Here's how the part is built. I have some questions about the finished solid (model axes, mm). Face numbers are marked on the shaded views. A direction names the side the tool comes from. Round coordinates to 2 decimals unless told otherwise and drop trailing zeros. Loops run counter-clockwise (first coordinate to the right, second up) from the corner with the lowest first, then second, coordinate; pieces in that order, holes last. Notation, with made-up numbers: (73, -29) -> (132, -29) arc R5 cw to (132, -20) -> close; hole circle Ø10 at (25.5, -23). An arc over 180 degrees is marked (long way). Use CSV: the item, a comma, the result in double quotes. Start each with the question number.
from build123d import *

# Parameters (mm, degrees)
BASE_FLANGE1_DEPTH      = 4.7752
EDGE_FLANGE1_DEPTH      = 50.8
EDGE_FLANGE1_BEND_DEPTH = 50.8
EDGE_FLANGE2_DEPTH      = 57.15
EDGE_FLANGE2_BEND_DEPTH = 57.15
CUT_EXTRUDE1_DEPTH      = 132.397433882
CUT_EXTRUDE1_DEPTH_BACK = 132.397433882
SKETCH18_R              = 5.159375
CUT_EXTRUDE3_DEPTH      = 122.772271015
CUT_EXTRUDE3_DEPTH_BACK = 122.772271015
SKETCH20_R              = 5.159375


# Sheet-metal steps are written as plain solids
with BuildPart() as part:
    # Sketch1 → Base-Flange1 (new body)
    with BuildSketch(Plane(origin=(0, 0, 0), x_dir=(1, 0, 0), z_dir=(0, 1, 0))):
        Polygon((26.9875, -28.575), (26.9875, 28.575), (28.575, 28.575), (28.575, 79.375), (-28.575, 79.375), (-28.575, -79.375), (28.575, -79.375), (28.575, -28.575), align=None)
    extrude(amount=-BASE_FLANGE1_DEPTH)

    # Edge-Flange1 section (across the edge) → Edge-Flange1 (add)
    with BuildSketch(Plane(origin=(34.5186, 0, -28.575), x_dir=(-1, 0, 0), z_dir=(0, 0, -1))):
        with BuildLine():
            Line((-4.7752, 5.9436), (-4.7752, 69.85))
            Line((-4.7752, 69.85), (0, 69.85))
            Line((0, 69.85), (0, 5.9436))
            ThreePointArc((0, 5.9436), (1.740840135, 1.740840135), (5.9436, 0))
            Line((5.9436, 0), (5.9436, -4.7752))
            ThreePointArc((5.9436, -4.7752), (-1.635736166, -1.635736166), (-4.7752, 5.9436))
        make_face()
    extrude(amount=EDGE_FLANGE1_DEPTH)

    # Edge-Flange1 section 2 (across the edge) → Edge-Flange1 bend (add)
    with BuildSketch(Plane(origin=(34.5186, 0, 79.375), x_dir=(-1, 0, 0), z_dir=(0, 0, -1))):
        with BuildLine():
            Line((-4.7752, 5.9436), (-4.7752, 69.85))
            Line((-4.7752, 69.85), (0, 69.85))
            Line((0, 69.85), (0, 5.9436))
            ThreePointArc((0, 5.9436), (1.740840135, 1.740840135), (5.9436, 0))
            Line((5.9436, 0), (5.9436, -4.7752))
            ThreePointArc((5.9436, -4.7752), (-1.635736166, -1.635736166), (-4.7752, 5.9436))
        make_face()
    extrude(amount=EDGE_FLANGE1_BEND_DEPTH)

    # Edge-Flange2 section (across the edge) → Edge-Flange2 (add)
    with BuildSketch(Plane(origin=(28.575, -4.7752, 86.9061), x_dir=(0, 0, -1), z_dir=(-1, 0, 0))):
        with BuildLine():
            Line((-4.7752, 5.9436), (-4.7752, 17.4498))
            Line((-4.7752, 17.4498), (0, 17.4498))
            Line((0, 17.4498), (0, 5.9436))
            ThreePointArc((0, 5.9436), (1.740840135, 1.740840135), (5.9436, 0))
            Line((5.9436, 0), (7.5311, 0))
            Line((7.5311, 0), (7.5311, -4.7752))
            Line((7.5311, -4.7752), (5.9436, -4.7752))
            ThreePointArc((5.9436, -4.7752), (-1.635736166, -1.635736166), (-4.7752, 5.9436))
        make_face()
    extrude(amount=EDGE_FLANGE2_DEPTH)

    # Edge-Flange2 section 2 (across the edge) → Edge-Flange2 bend (add)
    with BuildSketch(Plane(origin=(-28.575, -4.7752, -86.9061), x_dir=(0, 0, 1), z_dir=(1, 0, 0))):
        with BuildLine():
            Line((-4.7752, 5.9436), (-4.7752, 17.4498))
            Line((-4.7752, 17.4498), (0, 17.4498))
            Line((0, 17.4498), (0, 5.9436))
            ThreePointArc((0, 5.9436), (1.740840135, 1.740840135), (5.9436, 0))
            Line((5.9436, 0), (7.5311, 0))
            Line((7.5311, 0), (7.5311, -4.7752))
            Line((7.5311, -4.7752), (5.9436, -4.7752))
            ThreePointArc((5.9436, -4.7752), (-1.635736166, -1.635736166), (-4.7752, 5.9436))
        make_face()
    extrude(amount=EDGE_FLANGE2_BEND_DEPTH)

    # Sketch18 → Cut-Extrude1 (cut, two sides: drawn at the far end of the back side and taken through both)
    with BuildSketch(Plane.ZY.offset(-34.5186).offset(-CUT_EXTRUDE1_DEPTH_BACK)):
        with Locations(Location((-53.975, 50.8, 0), (0, 0, 270))):
            Circle(SKETCH18_R)
        with Locations(Location((-53.975, 19.05, 0), (0, 0, 270))):
            Circle(SKETCH18_R)
        with Locations(Location((53.975, 50.8, 0), (0, 0, 270))):
            Circle(SKETCH18_R)
        with Locations(Location((53.975, 19.05, 0), (0, 0, 270))):
            Circle(SKETCH18_R)
    extrude(amount=CUT_EXTRUDE1_DEPTH + CUT_EXTRUDE1_DEPTH_BACK, mode=Mode.SUBTRACT)

    # Sketch20 → Cut-Extrude3 (cut, two sides: drawn at the far end of the back side and taken through both)
    with BuildSketch(Plane(origin=(0, 0, 0), x_dir=(1, 0, 0), z_dir=(0, 1, 0)).offset(-CUT_EXTRUDE3_DEPTH_BACK)):
        with Locations((-72.900583951, 79.249926239)):
            Circle(SKETCH20_R)
        with Locations(Location((-3.175, 75.082739816, 0), (0, 0, 270))):
            Circle(SKETCH20_R)
        with Locations(Location((-9.236362071, -26.336291386, 0), (0, 0, 270))):
            Circle(SKETCH20_R)
        with Locations((-78.961946022, -22.169104962)):
            Circle(SKETCH20_R)
    extrude(amount=CUT_EXTRUDE3_DEPTH + CUT_EXTRUDE3_DEPTH_BACK, mode=Mode.SUBTRACT)


solid = part.part
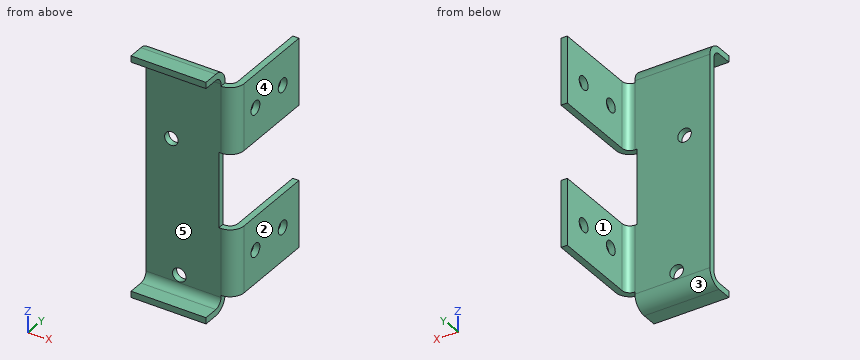
Q1. I want a section at C-C, the plane x = 7.5. List the corners of the cut face in (y, z) for me (1 decimal).
Q2. I want a section at D-D, the plane x = 30.5. List the corners of the cut face in (y, z) for me (3 decimals), then the cut area to 3 significant figures.
Q3. Will these pins go through, and if not, where does the flat tip stop? pin 1 Ø5 at (x, z) = (10, -22.5) entering from +Y; pin 2 Ø16.5 at (y, z) = (50.8, -53.975) entering from -X; pin 3 Ø3 at (x, y) = (3.5, -4.5) entering from -Z.
Q4. For the marked faces 1 and 2, which set-ups out of +Z, -Z, +X, -X, +Y, -Y let a thin tool reach every point of the face, with its end or its side?
Q5. I want a section at A-A, the plane y = 19.05. List the corners of the cut face in (x, z) for me (3 decimals), then the cut area to 3 significant figures.
Q6. I want a section at B-B, the plane z = -61.5. List the corners of the cut face in (x, y) for me (3 decimals), then the cut area to 3 significant figures.
Q7. I need wall thicknesses on line 1 along Z through (x, y) = (36.4, 50.8) (3 decimals); line 2 along Z through (x, y) = (11, -11); line 3 along Z through (x, y) = (37, 50) (3 decimals). Which ranges of each line are inside material? Lowest first, please.
Q8. If we mould it in two halves opening along Z, with no side actions, what happens to the marked faces 3, 4 and 5? For each: pulls with the +Z half, pulls with the -Z half, needs draft (parallel to the pull), parting line crosses it, or undercut.
Values found:
1,outline,"(-22.2, -91.7) -> (-10.7, -91.7) arc R10.7 ccw to (0, -81) -> (0, 81) arc R10.7 ccw to (-10.7, 91.7) -> (-22.2, 91.7) -> (-22.2, 86.9) -> (-10.7, 86.9) arc R5.9 cw to (-4.8, 81) -> (-4.8, -81) arc R5.9 cw to (-10.7, -86.9) -> (-22.2, -86.9) -> close"
2,outline,"(-4.601, -79.375) -> (0.32, -79.375) -> (0.32, -28.575) -> (-4.601, -28.575) -> close; (-4.601, 28.575) -> (0.32, 28.575) -> (0.32, 79.375) -> (-4.601, 79.375) -> close"
2,area,"500 mm2"
3,pin 1,"y = 0"
3,pin 2,"x = 34.52"
3,pin 3,"z = -90.59"
4,face 1,"+Z, -Z, -X, +Y"
4,face 2,"+Z, -Z, +X, +Y, -Y"
5,outline,"(34.519, -79.375) -> (39.294, -79.375) -> (39.294, -59.134) -> (34.519, -59.134) -> close; (34.519, -48.816) -> (39.294, -48.816) -> (39.294, -28.575) -> (34.519, -28.575) -> close; (34.519, 28.575) -> (39.294, 28.575) -> (39.294, 48.816) -> (34.519, 48.816) -> close; (34.519, 59.134) -> (39.294, 59.134) -> (39.294, 79.375) -> (34.519, 79.375) -> close"
5,area,"387 mm2"
6,outline,"(-28.575, -4.775) -> (28.575, -4.775) arc R10.719 ccw to (39.294, 5.944) -> (39.294, 69.85) -> (34.519, 69.85) -> (34.519, 5.944) arc R5.944 cw to (28.575, 0) -> (-28.575, 0) -> close"
6,area,"641 mm2"
7,line 1,"-79.375 to -59.134, -48.816 to -28.575, 28.575 to 48.816, 59.134 to 79.375"
7,line 2,"-91.68 to -86.91, 86.91 to 91.68"
7,line 3,"-79.375 to -59.072, -48.878 to -28.575, 28.575 to 48.878, 59.072 to 79.375"
8,face 3,"pulls with the -Z half"
8,face 4,"needs draft"
8,face 5,"undercut"
